Geometry check sheet. Reference: the model listing, model coordinates, mm. Face numbers are marked on the shaded views. A direction names the side the tool comes from. Round coordinates to 2 decimals unless told otherwise and drop trailing zeros. Order: outer loops, then holes, each group sorted by start corner. A loop starts at its lowest first (then second) coordinate and runs counter-clockwise, first axis right, second up. Notation, with made-up numbers: (67, 29) - (92, 29) arc R19 cw to (92, 42) - close; hole circle Ø9 at (23.25, 34). An arc over 180 degrees is marked (long way). One line per question, with ' | ' between items. Start each with the question number.
Q1. Tool access check on the marked faces 1, 2 and 3. Record the directions out of +Z, -Z, +X, -X, +Y, -Y that give a thin tool (end or side, any length) a straight path to the whole face; none if there is none.
Q2. Mould release check, pull along Z, two halves, no side actions. Record for the marked faces 4, 5, 6 and 7: +Z half, -Z half, draft (parallel to the pull), parting line (faces both ways), or undercut.
Q3. Sectioned sample at A-A, the plane x = 10. Enter the section's corners in (y, z), then the cut area to 3 significant figures.
Q4. Sectioned sample at C-C, the plane y = 21.5. Enter the section's corners in (x, z).
Q5. Sectioned sample at D-D, the plane z = 25. Enter the section's corners in (x, y), then the cut area to 3 significant figures.
Q6. Gauge pin test, flat ends, axial feed: P1, Ø18, axis at x = -47, z = 31.5, coming from the +Y side; P2, Ø3, axis at x = -77, y = -24.5, coming from the -Z side; P3, Ø24, axis at x = -67.5, y = 98.5, coming from the -Z side. Record the tip position at first contact, or that the pin passes through.
Q7. Sectioned sample at B-B, the plane z = 53. Enter the section's corners in (x, y), then the cut area to 3 significant figures.
Q8. Material ranges on line 1 along X through (y, z) = (119.5, 32.5); line 2 along Z through (x, y) = (-66.5, 127.5); line 3 along Y through (x, z) = (10, 48), recorded low to high.
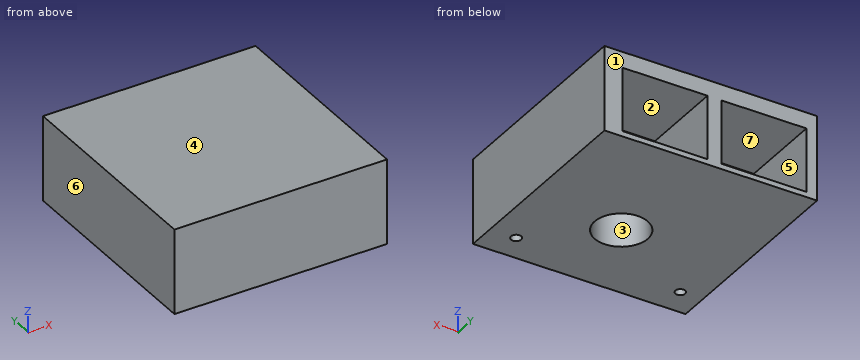
Autodesk Inventor part; units mm, degrees
ref_plane "YZ Plane" through (0, 0, 0) normal (1, 0, 0) x (0, 1, 0)
ref_plane "XZ Plane" through (0, 0, 0) normal (0, 1, 0) x (-1, 0, 0)
ref_plane "XY Plane" through (0, 0, 0) normal (0, 0, 1) x (1, 0, 0)
sketch "Sketch1" plane through (0, 0, 0) normal (0, 0, 1) x (1, 0, 0)
  line L0 (-100, -49.8579) -> (100, -49.8579)
  line L1 (100, -49.8579) -> (100, 150.1421)
  line L2 (100, 150.1421) -> (-100, 150.1421)
  line L3 (-100, 150.1421) -> (-100, -49.8579)
  line L4 (-100, -49.8579) -> (100, 150.1421) construction
  line L5 (100, -49.8579) -> (-100, 150.1421) construction
  point P0 (0, 50.1421)
  dimension "d13" = 200
  dimension "d14" = 200
  dimension "d17" = 200
extrude "Extrusion1" add sketch "Sketch1" along normal blind 80
sketch "Sketch2" plane through (-100, 150.1421, 0) normal (0, 1, 0) x (1, 0, 0)
  line L0 (90, -65) -> (10, -65)
  line L1 (10, -65) -> (10, -5)
  line L2 (10, -5) -> (90, -5)
  line L3 (90, -5) -> (90, -65)
  line L4 (90, -65) -> (10, -5) construction
  line L5 (10, -65) -> (90, -5) construction
  line L6 (0, 0) -> (0, -80)
  line L7 (200, 0) -> (0, 0)
  point P0 (100, 0)
  point P1 (50, -35)
  dimension "d7" = 80
  dimension "d8" = 60
  dimension "d9" = 10
  dimension "d10" = 5
extrude "Extrusion2" cut sketch "Sketch2" against normal blind 80
sketch "Sketch3" plane through (0, 0, 0) normal (0, 0, -1) x (-1, 0, 0)
  circle A0 centre (-10, 30.1421) radius 25
  line L0 (100, -49.8579) -> (-100, -49.8579)
  line L1 (-100, -49.8579) -> (-100, 150.1421)
  point P0 (0, 0)
  dimension "d19" = 50
  dimension "d20" = 80
  dimension "d21" = 90
extrude "Extrusion3" cut sketch "Sketch3" against normal blind 70
sketch "Sketch4" plane through (-100, 150.1421, 0) normal (0, 1, 0) x (1, 0, 0)
  line L0 (183.0719, -5) -> (103.0719, -5)
  line L1 (103.0719, -5) -> (103.0719, -65)
  line L2 (103.0719, -65) -> (183.0719, -65)
  line L3 (183.0719, -65) -> (183.0719, -5)
  line L4 (183.0719, -5) -> (103.0719, -65) construction
  line L5 (103.0719, -5) -> (183.0719, -65) construction
  line L6 (200, 0) -> (0, 0)
  point P0 (100, 0)
  point P1 (143.0719, -35)
  dimension "d24" = 80
  dimension "d25" = 60
  dimension "d26" = 5
extrude "Extrusion4" cut sketch "Sketch4" against normal blind 80
sketch "Sketch5" plane through (0, 0, 0) normal (0, 0, -1) x (-1, 0, 0)
  circle A0 centre (79.1012, -24.0908) radius 4.5958
  circle A1 centre (-75.3074, -24.0908) radius 4.8585
  point P0 (0, 0)
extrude "Extrusion5" cut sketch "Sketch5" against normal blind 45
properties part number "exploration1.1"
Determined:
1) face 1: +Z, -Z, +X, -X, +Y | face 2: +Y | face 3: -Z
2) face 4: +Z half | face 5: undercut | face 6: draft | face 7: undercut
3) outline: (-49.86, 0) - (5.14, 0) - (5.14, 70) - (55.14, 70) - (55.14, 0) - (150.14, 0) - (150.14, 5) - (70.14, 5) - (70.14, 65) - (150.14, 65) - (150.14, 80) - (-49.86, 80) - close | area: 7,700 mm2
4) outline: (-100, 0) - (-13.46, 0) - (-13.46, 70) - (33.46, 70) - (33.46, 0) - (100, 0) - (100, 80) - (-100, 80) - close
5) outline: (-100, -49.86) - (100, -49.86) - (100, 150.14) - (83.07, 150.14) - (83.07, 70.14) - (3.07, 70.14) - (3.07, 150.14) - (-10, 150.14) - (-10, 70.14) - (-90, 70.14) - (-90, 150.14) - (-100, 150.14) - close; hole circle Ø9.19 at (-79.1, -24.09); hole circle Ø50 at (10, 30.14); hole circle Ø9.72 at (75.31, -24.09) | area: 25,100 mm2
6) P1: stops at y = 70.14 | P2: stops at z = 45 | P3: stops at z = 0
7) outline: (-100, -49.86) - (100, -49.86) - (100, 150.14) - (83.07, 150.14) - (83.07, 70.14) - (3.07, 70.14) - (3.07, 150.14) - (-10, 150.14) - (-10, 70.14) - (-90, 70.14) - (-90, 150.14) - (-100, 150.14) - close; hole circle Ø50 at (10, 30.14) | area: 25,200 mm2
8) line 1: x = -100 to -90, -10 to 3.07, 83.07 to 100 | line 2: z = 0 to 5, 65 to 80 | line 3: y = -49.86 to 5.14, 55.14 to 70.14
